The model under review builds one solid part; all positions refer to its coordinate system, in mm. Face numbers are marked on the shaded views. Coordinates: 2 decimals unless noted, no trailing zeros. Loops run counter-clockwise (first coordinate to the right, second up) from the corner with the lowest first, then second, coordinate; pieces in that order, holes last. Notation, with made-up numbers: M 22,76.25 L 74,76.25 A14 ccw 74,80.25 Z; hole C -33,16 d4. An arc over 180 degrees is marked long. Use CSV: the item, a comma, the result in double quotes. Start each with the question number.
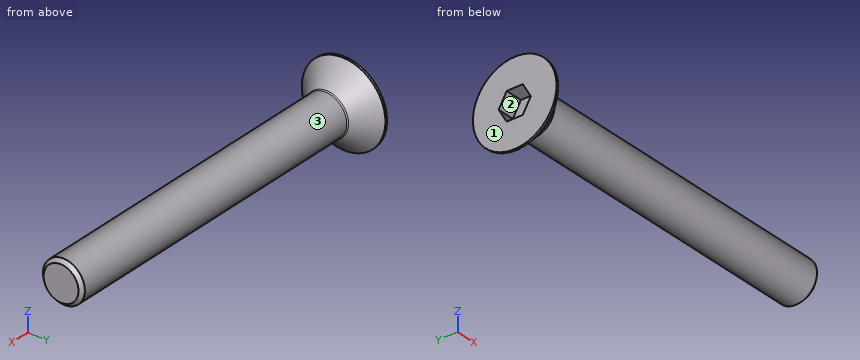
Autodesk Inventor part; units mm, degrees
ref_plane "MSC_PF1" through (0, 0, 0) normal (1, 0, 0) x (0, 1, 0)
ref_plane "MSC_PT1" through (0, 0, 0) normal (1, 0, 0) x (0, 1, 0)
ref_plane "YZ Plane" through (0, 0, 0) normal (1, 0, 0) x (0, 1, 0)
sketch "Skizze1" plane through (0, 0, 0) normal (0, 1, 0) x (-1, 0, 0)
  point P0 (0, 0)
sketch "Skizze2" plane through (0, 0, 0) normal (0, 0, 1) x (-1, 0, 0)
  line L0 (-50, 3) -> (-50, 0)
  line L1 (-3.3, 3) -> (-50, 3)
  line L2 (-0.3, 6) -> (-3.3, 3)
  line L3 (0, 6) -> (-0.3, 6)
  line L4 (0, 0) -> (0, 6)
  line L5 (-50, 0) -> (0, 0)
  line L6 (-50, 0) -> (0, 0)
  line L7 (0, -9.6) -> (0, 1.6)
  line L8 (10, 0) -> (-60, 0)
  dimension "ParC" = 0.3
  dimension "d43" = 45
  dimension "d44" = 6
  dimension "d45" = 3
  dimension "d46" = 50
  dimension "d47" = 0
  dimension "d48" = 0
revolve "Drehung1" add sketch "Skizze2" angle 360 about axis through (50, 0, 0) along (1, 0, 0)
sketch "Skizze3" plane through (0, 0, 0) normal (-1, 0, 0) x (0, 0, 1)
  line L0 (-2, 1.1547) -> (-2, -1.1547)
  line L1 (0, 2.3094) -> (-2, 1.1547)
  line L2 (2, 1.1547) -> (0, 2.3094)
  line L3 (2, -1.1547) -> (2, 1.1547)
  line L4 (0, -2.3094) -> (2, -1.1547)
  line L5 (-2, -1.1547) -> (0, -2.3094)
  circle A0 centre (0, 0) radius 2 construction
  circle A1 centre (0, 0) radius 3 construction
  dimension "d11" = 4
  dimension "d13" = 120
  dimension "d15" = 120
extrude "Extrusion1" cut sketch "Skizze3" against normal blind 2.5
fillet "Rundung1" radius 0.3 1 edges at (3.3, 3, 0)
chamfer "Fase1" distance 0.5 angle 45 1 edges at (50, 3, 0) measured on face at (34.4748, -2.4612, -1.7154)
thread "Gewinde1"
ref_plane "MSC_PF1" through (0, 0, 0) normal (1, 0, 0) x (0, 1, 0)
ref_plane "MSC_PT1" through (0, 0, 0) normal (1, 0, 0) x (0, 1, 0)
equation "\"d43\" = 0.5 * ang"
equation "\"d44\" = 0.5 * dk"
equation "\"d45\" = 0.5 * NND"
equation "\"d46\" = NLG"
equation "\"d11\" = ParS"
equation "\"d16\" = ParT"
equation "\"d18\" = r"
equation "\"d19\" = 0.5 * PTC"
equation "\"d39\" = 0.5 * PTC"
equation "\"NND\" = 6"
equation "\"PTC\" = 1"
equation "\"dk\" = 12"
equation "\"ParK\" = 3.3"
equation "\"ParS\" = 4"
equation "\"ParT\" = 2.5"
equation "\"r\" = 0.3"
equation "\"NLG\" = 50"
equation "\"ang\" = 90deg"
equation "\"THREADDIA\" = NND"
properties part number "ISO 10642 - M6 x  50" material "Stahl"
1. To check wall thickness, follow line 1 along X through (y, z) = (-2.5, 4.5); line 2 along Z through (x, y) = (26, 0); line 3 along X through (y, z) = (0.5, 1). State the ranges of each line that lie inside material, in increasing order.
2. Add section A-A (x = 11). Write out the cut boundary in (y, z).
3. Insertion check: pin 1 Ø6 at (x, y) = (26, 4) entering from -Z; pin 2 Ø0.7 at (x, y) = (1, 0.5) entering from -Z; pin 3 Ø2 at (x, z) = (31, 2) entering from -Y. Each pin has a flat end and moves straight along its axis. Give the tip position at first contact, or say it passes through.
4. Draft analysis for pull direction Y (two halves, no side actions). For the marked faces 1, 2 and 3, state which applies: released by +Y, released by -Y, zero draft, split by the parting line, or undercut.
Solved:
1,line 1,"x = 0 to 1.15"
1,line 2,"z = -3 to 3"
1,line 3,"x = 2.5 to 50"
2,outline,"C 0,0 d6"
3,pin 1,"stops at z = -2.83"
3,pin 2,"stops at z = -5.63"
3,pin 3,"stops at y = -2.83"
4,face 1,"zero draft"
4,face 2,"undercut"
4,face 3,"split by the parting line"
